```python
from build123d import *

# Parameters (mm, degrees)
F0_R     = 4.25
F1_DEPTH = 3
F2_START = 3
F2_DEPTH = 2
F3_START = 5
F3_DEPTH = 10


with BuildPart() as f1:
    # F0 (on Top) → F1 (new body)
    with BuildSketch(Plane.XY):
        Circle(F0_R)
        with BuildLine():
            ThreePointArc((1.65, 2.1371710273), (2.4233241632, 1.19058809), (2.7, 0))
            ThreePointArc((2.7, 0), (2.4233241632, -1.19058809), (1.65, -2.1371710273))
            ThreePointArc((1.65, -2.1371710273), (0, -2.7), (-1.65, -2.1371710273))
            ThreePointArc((-1.65, -2.1371710273), (-2.7, 0), (-1.65, 2.1371710273))
            ThreePointArc((-1.65, 2.1371710273), (0, 2.7), (1.65, 2.1371710273))
        make_face(mode=Mode.SUBTRACT)
    extrude(amount=F1_DEPTH)

    # F0 (on Top) → F2 (join)
    with BuildSketch(Plane.XY.offset(F2_START)):
        Circle(F0_R)
        with BuildLine():
            ThreePointArc((1.65, 2.1371710273), (2.4233241632, 1.19058809), (2.7, 0))
            ThreePointArc((2.7, 0), (2.4233241632, -1.19058809), (1.65, -2.1371710273))
            ThreePointArc((1.65, -2.1371710273), (0, -2.7), (-1.65, -2.1371710273))
            ThreePointArc((-1.65, -2.1371710273), (-2.7, 0), (-1.65, 2.1371710273))
            ThreePointArc((-1.65, 2.1371710273), (0, 2.7), (1.65, 2.1371710273))
        make_face(mode=Mode.SUBTRACT)
        with BuildLine():
            Line((-1.65, -2.1371710273), (-1.65, 2.1371710273))
            ThreePointArc((-1.65, 2.1371710273), (-2.7, 0), (-1.65, -2.1371710273))
        make_face()
        with BuildLine():
            ThreePointArc((1.65, -2.1371710273), (2.4233241632, -1.19058809), (2.7, 0))
            ThreePointArc((2.7, 0), (2.4233241632, 1.19058809), (1.65, 2.1371710273))
            Line((1.65, 2.1371710273), (1.65, -2.1371710273))
        make_face()
    extrude(amount=F2_DEPTH)

    # F0 (on Top) → F3 (join)
    with BuildSketch(Plane.XY.offset(F3_START)):
        Polygon((-6.625094339, -3.825), (0, -7.65), (6.625094339, -3.825), (6.625094339, 3.825), (0, 7.65), (-6.625094339, 3.825), align=None)
        Circle(F0_R, mode=Mode.SUBTRACT)
        Circle(F0_R)
        with BuildLine():
            ThreePointArc((1.65, 2.1371710273), (2.4233241632, 1.19058809), (2.7, 0))
            ThreePointArc((2.7, 0), (2.4233241632, -1.19058809), (1.65, -2.1371710273))
            ThreePointArc((1.65, -2.1371710273), (0, -2.7), (-1.65, -2.1371710273))
            ThreePointArc((-1.65, -2.1371710273), (-2.7, 0), (-1.65, 2.1371710273))
            ThreePointArc((-1.65, 2.1371710273), (0, 2.7), (1.65, 2.1371710273))
        make_face(mode=Mode.SUBTRACT)
        with BuildLine():
            ThreePointArc((1.65, -2.1371710273), (2.4233241632, -1.19058809), (2.7, 0))
            ThreePointArc((2.7, 0), (2.4233241632, 1.19058809), (1.65, 2.1371710273))
            Line((1.65, 2.1371710273), (1.65, -2.1371710273))
        make_face()
        with BuildLine():
            Line((-1.65, -2.1371710273), (-1.65, 2.1371710273))
            ThreePointArc((-1.65, 2.1371710273), (-2.7, 0), (-1.65, -2.1371710273))
        make_face()
    extrude(amount=F3_DEPTH)

    # F4 (on Right) → F5 (revolve, cut)
    with BuildSketch(Plane.YZ):
        Polygon((-8.316071704, 4.8156171106), (-6.5929647535, 15.9113816917), (-8.316071704, 15.9113816917), align=None)
    revolve(axis=Axis((0, 0, 4.9219373614), (0, 0, 1)), mode=Mode.SUBTRACT)


solid = f1.part
```
Could you check a few things on this model? Use its own coordinates, in mm. A direction names the side the tool comes from. Round coordinates to 2 decimals unless told otherwise and drop trailing zeros. Write each loop counter-clockwise with the first axis right and the second up, starting at its lowest first coordinate (ties: lowest second). Pieces come first, ordered by that corner, then holes.
(1) Suppose I cut it at B-B on z = 7. Write out the boundary of the cut face in (x, y) (3 decimals), and give its area (3 significant figures).
Findings below:
outline: (-6.625, -3.825) - (0, -7.65) - (6.625, -3.825) - (6.625, 3.825) - (0, 7.65) - (-6.625, 3.825) - close; hole (-1.65, -2.137) arc R2.7 ccw to (1.65, -2.137) - (1.65, 2.137) arc R2.7 ccw to (-1.65, 2.137) - close
area: 135 mm2
(2) If I drill on probe 1 along X at (y, z) = (0, 11); probe 2 along Y at (x, z) = (0, 4), over which ranges is the centre line in solid material (lowest first)?
Findings below:
probe 1: x = -6.63 to -1.65, 1.65 to 6.63
probe 2: y = -4.25 to -2.7, 2.7 to 4.25
(3) Which directions (+Z, -Z, +X, -X, +Y, -Y) give clear straight access to the entire face, cutting with the end or side of a thin tool? Please do faces 1 (the face through (1.65, 0, 9)), 2 (the face through (-3, -3.3, 5)), 3 (the face through (0.034, 6.982, 13.404)).
Findings below:
face 1: +Z, -Z
face 2: -Z
face 3: +Z, +Y
(4) Suppose I cut it at D-D on x = 3.5. Write out the boundary of the cut face in (y, z), and give its area (3 significant figures).
Findings below:
outline: (-5.63, 5) - (-2.41, 5) - (-2.41, 0) - (2.41, 0) - (2.41, 5) - (5.63, 5) - (5.63, 15) - (-5.63, 15) - close
area: 137 mm2
(5) Suppose I cut it at A-A on y = 0. Write out the boundary of the cut face in (x, z), and give its area (3 significant figures).
Findings below:
outline: (-6.63, 5) - (-4.25, 5) - (-4.25, 0) - (-2.7, 0) - (-2.7, 3) - (-1.65, 3) - (-1.65, 15) - (-6.63, 15) - close; (1.65, 3) - (2.7, 3) - (2.7, 0) - (4.25, 0) - (4.25, 5) - (6.63, 5) - (6.63, 15) - (1.65, 15) - close
area: 119 mm2
(6) Thinking about a two-plate mould opening in X: for faces 4 (the face through (3.27, -5.76, 8.82)), 5 (the face through (-0.034, -6.982, 13.404)), 6 (the face through (1.13, -2.45, 5.73)), 7 (the face through (-6.064, -3.462, 13.404)), which applies, +X half, -X half, draft (parallel to the pull), parting line (faces both ways), or undercut?
Findings below:
face 4: +X half
face 5: parting line
face 6: undercut
face 7: -X half
(7) For pin 1 (5 mm diameter, centred on y = 3.5, z = 11.5, fed in from -X); pin 2 (1 mm diameter, centred on y = -6, z = 9.5, fed in from +X); pin 3 (3 mm diameter, centred on y = 0.5, z = 2.5, fed in from -X), each with a flat end and sliding along its axis, tell me the tip position at first contact or that it passes through.
Findings below:
pin 1: stops at x = -6.63
pin 2: stops at x = 3.72
pin 3: stops at x = -4.25
(8) Suppose I cut it at C-C on z = 13.25. Write out the boundary of the cut face in (x, y), and give its area (3 significant figures).
Findings below:
outline: (-6.63, -2.28) arc R7.01 ccw to (-5.29, -4.6) - (-1.34, -6.88) arc R7.01 ccw to (1.34, -6.88) - (5.29, -4.6) arc R7.01 ccw to (6.63, -2.28) - (6.63, 2.28) arc R7.01 ccw to (5.29, 4.6) - (1.34, 6.88) arc R7.01 ccw to (-1.34, 6.88) - (-5.29, 4.6) arc R7.01 ccw to (-6.63, 2.28) - close; hole (-1.65, -2.14) arc R2.7 ccw to (1.65, -2.14) - (1.65, 2.14) arc R2.7 ccw to (-1.65, 2.14) - close
area: 131 mm2
